Design review of the part shown in the three views and the two pictorial views. Dimensions are in mm from the part's minimum x, y and z. A direction names the side the tool comes from. Round coordinates to 2 decimals unless told otherwise and drop trailing zeros. Loops run counter-clockwise (first coordinate to the right, second up) from the corner with the lowest first, then second, coordinate; pieces in that order, holes last. Notation, with made-up numbers: (61.25, 63.5) -> (70.25, 63.5) arc R6 cw to (70.25, 71.5) -> close; hole circle Ø8 at (-38, -35). An arc over 180 degrees is marked (long way). Use a Markdown table: item, result. Add a question column.
1) Mouldability with a two-part tool opening along Y and no side actions: class the marked faces 1, 2, 3 and 4 as released by +Y, released by -Y, zero draft, split by the parting line, or undercut.
2) Wall thickness on probe 1 along Y at (x, z) = (4.5, 5) (1 decimal); probe 2 along Y at (x, z) = (1.6, 3) (1 decimal); probe 3 along Z at (x, y) = (0.7, 6.25): over which ranges is each line inside the solid? List them lowest first.
3) Insertion check: pin 1 (2 mm diameter, centred on x = 0.5, z = 2, fed in from -Y) (1 decimal); pin 2 (2 mm diameter, centred on x = 2.5, z = 3, fed in from +Y); pin 3 (1.5 mm diameter, centred on y = 2.5, z = 7.5, fed in from -X). Each pin has a flat end and moves straight along its axis. Give the tip position at first contact, or say it passes through.
4) Consider section A-A on x = 4.4. Give the boundary of the cut face in (y, z).
5) For the marked faces 5 and 6, list the 3-axis set-ups (+Z, -Z, +X, -X, +Y, -Y) from which the entire face can be reached by the end or side of a thin tool; tool diameter is ignored.
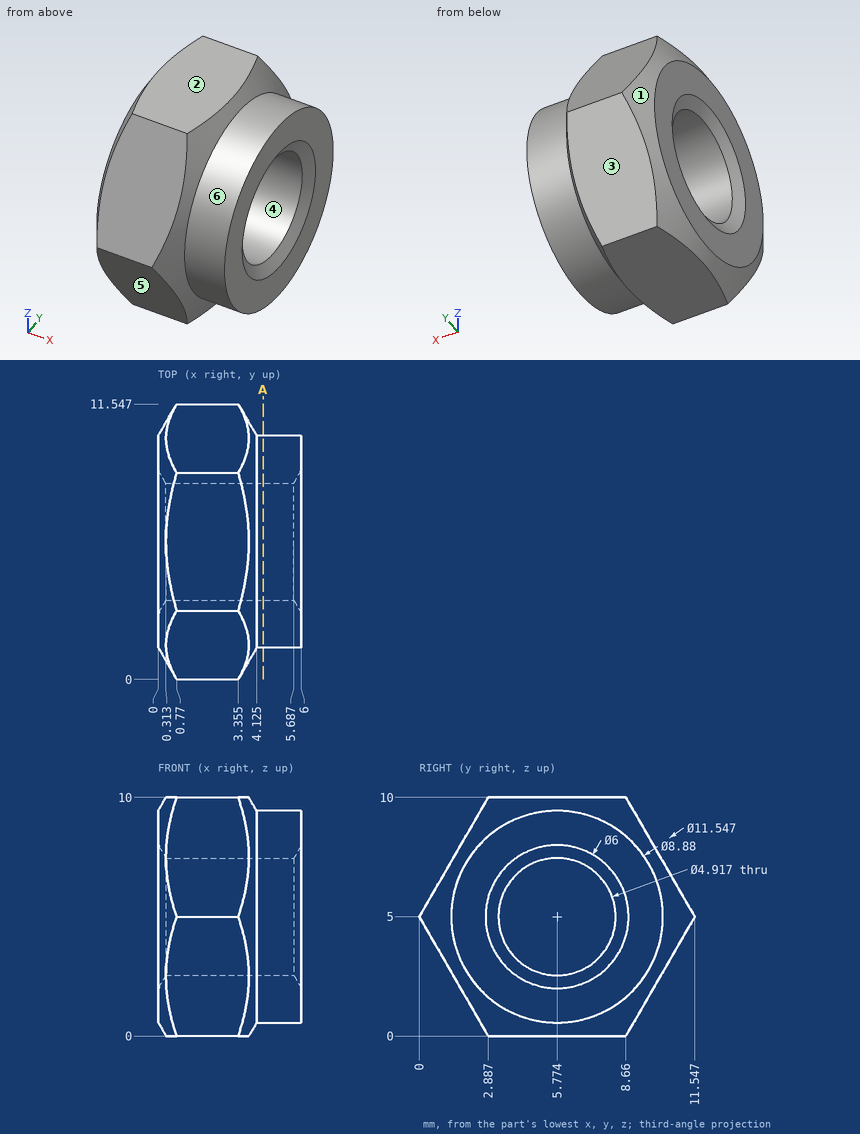
Result set:
| question | item | result |
|---|---|---|
| 1 | face 1 | split by the parting line |
| 1 | face 2 | zero draft |
| 1 | face 3 | released by +Y |
| 1 | face 4 | undercut |
| 2 | probe 1 | 1.3 to 3.3, 8.2 to 10.2 |
| 2 | probe 2 | 1.2 to 4.3, 7.2 to 10.4 |
| 2 | probe 3 | 0 to 2.59, 7.41 to 10 |
| 3 | pin 1 | y = 1.2 |
| 3 | pin 2 | y = 10.97 |
| 3 | pin 3 | x = 0 |
| 4 | outline | circle Ø8.88 at (5.77, 5); hole circle Ø4.92 at (5.77, 5) |
| 5 | face 5 | -Z, +X, -X, -Y |
| 5 | face 6 | +X |
